The listing builds one solid part. Answer for the finished solid, in the listing's coordinates (mm). A direction names the side the tool comes from. Give positions to 0.01 mm unless a question says otherwise; leave off trailing zeros. Loops run counter-clockwise (first coordinate to the right, second up) from the corner with the lowest first, then second, coordinate; pieces in that order, holes last. Notation, with made-up numbers: M 7.25,21.25 L 59.25,21.25 A32 ccw 59.25,47.25 Z; hole C -35.75,18 d3. An arc over 180 degrees is marked long. Use one line per item in the form item = value. Start each with the question number.
1. The part is cut by section B-B (y = 1.5). Write down the section's boundary in (x, z).
2. The mould has two halves that part along X. Classify faces 1 (the face through (6, 0, -4)), 2 (the face through (-2, 2, -5.5)), 3 (the face through (2.44, -0.54, -2.2)): released by +X, released by -X, zero draft, split by the parting line, or undercut.
3. The part is cut by section D-D (y = 3). Write down the section's boundary in (x, z), and give its area (3 significant figures).
4. Straight lines are drawn through the part: line 1 (Y direction, x = 0, z = -0.75); line 2 (Y direction, x = -1.25, z = -1.25); line 3 (Z direction, x = 5.5, y = 6). For each, find the intervals that lie inside material, in ascending order. Write a range as from..to.
5. Each of these flat-tipped pins is pushed along its axis until it touches: pin 1 Ø0.6 at (y, z) = (1, 0.5) entering from -X; pin 2 Ø6.5 at (x, y) = (0, 0) entering from +Z; pin 3 Ø1 at (y, z) = (1.5, -4.5) entering from +X. Where does it stop, or does it pass through?
6. For faces 4 (the face through (6, 0, 0)), 5 (the face through (-6, 0, 0)), 6 (the face through (0, 7, -2)), determine the directions among +Z, -Z, +X, -X, +Y, -Y from which every point of the face is accessible in a straight line to the end or side of a thin tool.
7. The part is cut by section A-A (x = 1.5). Write down the section's boundary in (y, z).
8. The part is cut by section C-C (z = -3). Write down the section's boundary in (x, y).
from build123d import *

# Parameters (mm, degrees)
SKETCH1_W      = 15
SKETCH1_H      = 14
EXTRUDE1_DEPTH = 5.5
SKETCH2_W      = 7.8
SKETCH2_H      = 14
EXTRUDE2_DEPTH = 1
SKETCH7_W      = 2.5
SKETCH7_H      = 6.500025
CHAMFER1_SIZE  = 3
FILLET1_R      = 0.3


with BuildPart() as part:
    # Sketch1 → Extrude1 (new body)
    with BuildSketch(Plane.XY):
        Rectangle(SKETCH1_W, SKETCH1_H)
    extrude(amount=-EXTRUDE1_DEPTH)

    # Sketch2 → Extrude2 (add)
    with BuildSketch(Plane.XY):
        Rectangle(SKETCH2_W, SKETCH2_H)
    extrude(amount=EXTRUDE2_DEPTH)

    # Sketch7 → M6x1.0 Tapped Hole1 (revolve, cut)
    with BuildSketch(Plane(origin=(0, 0, -5.5), x_dir=(0, 1, 0), z_dir=(1, 0, 0))):
        with Locations((1.25, 3.2500125)):
            Rectangle(SKETCH7_W, SKETCH7_H)
    revolve(axis=Axis((0, 0, -11.85), (0, 0, 1)), mode=Mode.SUBTRACT)

    # Chamfer1
    chamfer1_edges = [part.edges().sort_by_distance(p)[0] for p in [
        (7.5, 0, -5.5),
        (-7.5, 0, -5.5),
    ]]
    chamfer(chamfer1_edges, length=CHAMFER1_SIZE)

    # Fillet1
    fillet1_edges = [part.edges().sort_by_distance(p)[0] for p in [
        (-3.9, 0, 0),
        (3.9, 0, 0),
        (7.5, 0, -2.5),
        (-7.5, 0, -2.5),
    ]]
    fillet(fillet1_edges, radius=FILLET1_R)


solid = part.part
Derived:
q1.outline = M -7.5,-2.38 A0.3 ccw -7.41,-2.59 L -4.5,-5.5 L -2,-5.5 L -2,1 L -3.9,1 L -3.9,0.3 A0.3 cw -4.2,0 L -7.5,0 Z; M 2,-5.5 L 4.5,-5.5 L 7.41,-2.59 A0.3 ccw 7.5,-2.38 L 7.5,0 L 4.2,0 A0.3 cw 3.9,0.3 L 3.9,1 L 2,1 Z
q2.face_1 = released by +X
q2.face_2 = zero draft
q2.face_3 = undercut
q3.outline = M -7.5,-2.38 A0.3 ccw -7.41,-2.59 L -4.5,-5.5 L 4.5,-5.5 L 7.41,-2.59 A0.3 ccw 7.5,-2.38 L 7.5,0 L 4.2,0 A0.3 cw 3.9,0.3 L 3.9,1 L -3.9,1 L -3.9,0.3 A0.3 cw -4.2,0 L -7.5,0 Z
q3.area = 81.3 mm2
q4.line_1 = -7..-2.5, 2.5..7
q4.line_2 = -7..-2.17, 2.17..7
q4.line_3 = -4.5..0
q5.pin_1 = -3.92
q5.pin_2 = 1
q5.pin_3 = 6
q6.face_4 = +Z, +X, +Y, -Y
q6.face_5 = +Z, -X, +Y, -Y
q6.face_6 = +Z, -Z, +X, -X, +Y
q7.outline = M -7,-5.5 L -2,-5.5 L -2,1 L -7,1 Z; M 2,-5.5 L 7,-5.5 L 7,1 L 2,1 Z
q8.outline = M -7,-7 L 7,-7 L 7,7 L -7,7 Z; hole C 0,0 d5
